```python
from build123d import *

# Parameters (mm, degrees)
SKETCH_R  = 1.75
PAD_DEPTH = 5


with BuildPart() as part:
    # Sketch → Pad (new body)
    with BuildSketch(Plane.XY):
        with BuildLine():
            ThreePointArc((0, 5), (-5, 0), (0, -5))
            Line((0, -5), (266, -5))
            ThreePointArc((266, -5), (271, 0), (266, 5))
            Line((266, 5), (0, 5))
        make_face()
        Circle(SKETCH_R, mode=Mode.SUBTRACT)
        with Locations((266, 0)):
            Circle(SKETCH_R, mode=Mode.SUBTRACT)
        with Locations((133, 0)):
            Circle(SKETCH_R, mode=Mode.SUBTRACT)
    extrude(amount=PAD_DEPTH)


solid = part.part
```
Build history of the part. All positions in model axes, mm. Round coordinates to 2 decimals unless told otherwise and drop trailing zeros. Loops run counter-clockwise (first coordinate to the right, second up) from the corner with the lowest first, then second, coordinate; pieces in that order, holes last.
Item 1: Pin check, flat tips, straight feed: P1, Ø2, axis at x = 120.5, y = 3.5, coming from the -Z side; P2, Ø3, axis at x = 133, y = 0, coming from the -Z side. Stop position of each tip, or through.
Item 2: Saw through at A-A (y = 0). List the corners of the cut face in (x, z), then the cut area to 3 significant figures.
Item 3: Drill centre lines: line 1 along X through (y, z) = (0.25, 3.9); line 2 along Y through (x, z) = (0, 1.35); line 3 along X through (y, z) = (-1, 3.35). Where is each one in solid material? Low to high.
Item 4: Saw through at B-B (z = 1.85). List the corners of the cut face in (x, y).
Worked answers:
1. P1: stops at z = 0
1. P2: passes through
2. outline: (-5, 0) - (-1.75, 0) - (-1.75, 5) - (-5, 5) - close; (1.75, 0) - (131.25, 0) - (131.25, 5) - (1.75, 5) - close; (134.75, 0) - (264.25, 0) - (264.25, 5) - (134.75, 5) - close; (267.75, 0) - (271, 0) - (271, 5) - (267.75, 5) - close
2. area: 1,330 mm2
3. line 1: x = -4.99 to -1.73, 1.73 to 131.27, 134.73 to 264.27, 267.73 to 270.99
3. line 2: y = -5 to -1.75, 1.75 to 5
3. line 3: x = -4.9 to -1.44, 1.44 to 131.56, 134.44 to 264.56, 267.44 to 270.9
4. outline: (0, -5) - (266, -5) arc R5 ccw to (266, 5) - (0, 5) arc R5 ccw to start; hole circle Ø3.5 at (0, 0); hole circle Ø3.5 at (133, 0); hole circle Ø3.5 at (266, 0)
